```python
from build123d import *

# Parameters (mm, degrees)
SKETCH1_W           = 20
SKETCH1_H           = 20
BOSS_EXTRUDE1_DEPTH = 200
SKETCH2_W           = 10
SKETCH2_H           = 20
CUT_EXTRUDE1_DEPTH  = 21
SKETCH3_W           = 6.25
SKETCH3_H           = 6.25
CUT_EXTRUDE2_DEPTH  = 21
SKETCH4_W           = 6.25
SKETCH4_H           = 6.25
CUT_EXTRUDE3_DEPTH  = 21
SKETCH5_W           = 10
SKETCH5_H           = 15
CUT_EXTRUDE4_DEPTH  = 21


with BuildPart() as part:
    # Sketch1 → Boss-Extrude1 (new body)
    with BuildSketch(Plane(origin=(0, 0, 0), x_dir=(1, 0, 0), z_dir=(0, 1, 0))):
        with Locations((10, 10)):
            Rectangle(SKETCH1_W, SKETCH1_H)
    extrude(amount=BOSS_EXTRUDE1_DEPTH)

    # Sketch2 → Cut-Extrude1 (cut, through all)
    with BuildSketch(Plane(origin=(20, 0, 0), x_dir=(0, 0, -1), z_dir=(1, 0, 0))):
        with Locations((5, 190)):
            Rectangle(SKETCH2_W, SKETCH2_H)
        with Locations((5, 10)):
            Rectangle(SKETCH2_W, SKETCH2_H)
    extrude(amount=-CUT_EXTRUDE1_DEPTH, mode=Mode.SUBTRACT)

    # Sketch3 → Cut-Extrude2 (cut, through all)
    with BuildSketch(Plane(origin=(0, 0, -20), x_dir=(-1, 0, 0), z_dir=(0, 0, -1))):
        with Locations((-3.125, 196.875)):
            Rectangle(SKETCH3_W, SKETCH3_H)
        with Locations((-16.875, 196.875)):
            Rectangle(SKETCH3_W, SKETCH3_H)
        with Locations((-16.875, 183.125)):
            Rectangle(SKETCH3_W, SKETCH3_H)
        with Locations((-3.125, 183.125)):
            Rectangle(SKETCH3_W, SKETCH3_H)
    extrude(amount=-CUT_EXTRUDE2_DEPTH, mode=Mode.SUBTRACT)

    # Sketch4 → Cut-Extrude3 (cut, through all)
    with BuildSketch(Plane(origin=(0, 0, -20), x_dir=(-1, 0, 0), z_dir=(0, 0, -1))):
        with Locations((-16.875, 16.875)):
            Rectangle(SKETCH4_W, SKETCH4_H)
        with Locations((-16.875, 3.125)):
            Rectangle(SKETCH4_W, SKETCH4_H)
        with Locations((-3.125, 16.875)):
            Rectangle(SKETCH4_W, SKETCH4_H)
        with Locations((-3.125, 3.125)):
            Rectangle(SKETCH4_W, SKETCH4_H)
    extrude(amount=-CUT_EXTRUDE3_DEPTH, mode=Mode.SUBTRACT)

    # Sketch5 → Cut-Extrude4 (cut, through all)
    with BuildSketch(Plane.XY):
        with Locations((10, 40)):
            Rectangle(SKETCH5_W, SKETCH5_H)
        with Locations((10, 60)):
            Rectangle(SKETCH5_W, SKETCH5_H)
        with Locations((10, 80)):
            Rectangle(SKETCH5_W, SKETCH5_H)
        with Locations((10, 100)):
            Rectangle(SKETCH5_W, SKETCH5_H)
        with Locations((10, 120)):
            Rectangle(SKETCH5_W, SKETCH5_H)
        with Locations((10, 140)):
            Rectangle(SKETCH5_W, SKETCH5_H)
        with Locations((10, 160)):
            Rectangle(SKETCH5_W, SKETCH5_H)
    extrude(amount=-CUT_EXTRUDE4_DEPTH, mode=Mode.SUBTRACT)


solid = part.part
```
Part model, mm, in its own coordinate system. A direction names the side the tool comes from. Give positions to 0.01 mm unless a question says otherwise; leave off trailing zeros. Order: outer loops, then holes, each group sorted by start corner. A loop starts at its lowest first (then second) coordinate and runs counter-clockwise, first axis right, second up. Notation, with made-up numbers: M 19,52 L 50,52 A30 ccw 50,88 Z; hole C 67,41 d7. An arc over 180 degrees is marked long. Use a Markdown table: item, result. Add a question column.
(1) Mould opens along X. For faces 1 (the face through (6.25, 183, -15)), 2 (the face through (15, 60, -10)), 3 (the face through (3, 13.75, -15)) say: +X half, -X half, draft (parallel to the pull), parting line (faces both ways), or undercut.
(2) Saw through at B-B, the plane y = 77. Give the cut face in (x, z), and give its area (3 significant figures).
(3) Drop flat-ended pins along their axis: P1, Ø5, axis at x = 9.5, z = -7, coming from the +Y side; P2, Ø1.5, axis at x = 16.5, z = -10.5, coming from the -Y side. Give the stop position or say it passes through.
(4) Saw through at A-A, the plane x = 3.25. Give the cut face in (y, z), and give its area (3 significant figures).
(5) Probe line 1 along Y through (x, z) = (15.5, -17.25); line 2 along X through (y, z) = (138, -17.25); line 3 along Y through (x, z) = (18, -9.5). List the from-to ranges inside material, lowest first. Write a range as [from, to].
(6) Saw through at C-C, the plane z = -2.75. Give the number of separate pieces and of enclosed holes in the cut face, and give its area (3 significant figures).
(7) 3-axis set-ups, long thin cutter, end or side, ignore diameter. For faces 4 (the face through (10, 167.5, -10)), 5 (the face through (3, 99, 0)), 6 (the face through (13.75, 197, -15)), 7 (the face through (6.25, 197, -15)): which of +Z, -Z, +X, -X, +Y, -Y reach the whole face in a straight line?
Answer key:
| question | item | result |
|---|---|---|
| 1 | face 1 | -X half |
| 1 | face 2 | undercut |
| 1 | face 3 | draft |
| 2 | outline | M 0,-20 L 5,-20 L 5,0 L 0,0 Z; M 15,-20 L 20,-20 L 20,0 L 15,0 Z |
| 2 | area | 200 mm^2 |
| 3 | P1 | y = 180 |
| 3 | P2 | y = 6.25 |
| 4 | outline | M 6.25,-20 L 13.75,-20 L 13.75,-10 L 6.25,-10 Z; M 20,-20 L 180,-20 L 180,0 L 20,0 Z; M 186.25,-20 L 193.75,-20 L 193.75,-10 L 186.25,-10 Z |
| 4 | area | 3,350 mm^2 |
| 5 | line 1 | [6.25, 13.75], [20, 180], [186.25, 193.75] |
| 5 | line 2 | [0, 5], [15, 20] |
| 5 | line 3 | [20, 180] |
| 6 | separate pieces | 1 |
| 6 | enclosed holes | 7 |
| 6 | area | 2,150 mm^2 |
| 7 | face 4 | +Z, -Z |
| 7 | face 5 | +Z, +X, -X, +Y, -Y |
| 7 | face 6 | +Z, -Z, +X, +Y |
| 7 | face 7 | +Z, -Z, -X, +Y |
